Autodesk Inventor part; units mm, degrees
ref_plane "HF-Kabel-DurchlassPunkt" through (-139.5, -56.5, 0) normal (0, -1, 0) x (1, 0, 0)
ref_plane "YZ Plane" through (0, 0, 0) normal (1, 0, 0) x (0, 1, 0)
ref_plane "XZ Plane" through (0, 0, 0) normal (0, 1, 0) x (-1, 0, 0)
sketch "Skizze1" plane through (0, 0, 0) normal (0, 0, 1) x (1, 0, 0)
  line L0 (-149.5, 270.5) -> (149.5, 270.5)
  line L1 (149.5, 270.5) -> (149.5, -270.5)
  line L2 (149.5, -270.5) -> (-149.5, -270.5)
  line L3 (-149.5, -270.5) -> (-149.5, 270.5)
  line L4 (-149.5, 270.5) -> (149.5, -270.5) construction
  line L5 (149.5, 270.5) -> (-149.5, -270.5) construction
  line L6 (-74.75, 270.5) -> (-74.75, -270.5) construction
  line L7 (0, 396.7) -> (0, -381.7) construction
  line L8 (-142.5, 270.5) -> (-142.5, -270.5) construction
  line L9 (-149.5, -162.3) -> (149.5, -162.3) construction
  circle A0 centre (-142.5, -154.8) radius 3.25
  circle A1 centre (-142.5, -169.8) radius 3.25
  line L10 (-222.3, 0) -> (287.3, 0) construction
  circle A2 centre (-142.5, 7.5) radius 3.25
  circle A3 centre (-142.5, -7.5) radius 3.25
  circle A4 centre (-142.5, 154.8) radius 3.25
  circle A5 centre (-142.5, 169.8) radius 3.25
  circle A6 centre (142.5, -154.8) radius 3.25
  circle A7 centre (142.5, -169.8) radius 3.25
  circle A8 centre (142.5, 7.5) radius 3.25
  circle A9 centre (142.5, -7.5) radius 3.25
  circle A10 centre (142.5, 169.8) radius 3.25
  circle A11 centre (142.5, 154.8) radius 3.25
  circle A12 centre (-60, -162.3) radius 2.75
  circle A13 centre (60, -162.3) radius 2.75
  circle A14 centre (-60, 162.3) radius 2.75
  circle A15 centre (60, 162.3) radius 2.75
  line L11 (214.5, 285.5) -> (84.5, 285.5) construction
  line L12 (84.5, 285.5) -> (84.5, 255.5)
  line L13 (84.5, 255.5) -> (214.5, 255.5)
  line L14 (214.5, 255.5) -> (214.5, 285.5) construction
  line L15 (214.5, 285.5) -> (84.5, 255.5) construction
  line L16 (84.5, 285.5) -> (214.5, 255.5) construction
  point P0 (0, 0)
  dimension "d0" = 541
  dimension "d1" = 299
  dimension "d2" = 74.75
  dimension "d3" = 7
  dimension "d4" = 108.2
  dimension "d5" = 6.5
  dimension "d6" = 7.5
  dimension "d7" = 6.5
  dimension "d8" = 7.5
  dimension "d9" = 7.5
  dimension "d10" = 6.5
  dimension "d11" = 5.5
  dimension "d12" = 60
  dimension "d15" = 130
  dimension "d16" = 15
extrude "Extrusion1" add sketch "Skizze1" along normal blind 3
chamfer "Fase1" distance 10 angle 45 4 edges at (149.5, 270.5, 1.5) (149.5, -270.5, 1.5) (-149.5, -270.5, 1.5) (-149.5, 270.5, 1.5)
ref_plane "HF-Kabel-DurchlassPunkt" through (-139.5, -56.5, 0) normal (0, -1, 0) x (1, 0, 0)
sketch "S-AussparungHFKabel" plane through (0, 0, 3) normal (0, 0, 1) x (1, 0, 0)
  line L0 (209.3, -56.5) -> (-209.3, -56.5) construction
  line L1 (-149.5, 260.5) -> (-149.5, -260.5)
  line L2 (-149.5, -75) -> (-129.5, -63.453)
  line L3 (-129.5, -63.453) -> (-129.5, 63.453)
  line L4 (-129.5, 63.453) -> (-149.5, 75)
  line L5 (-129.5, 0) -> (-149.5, 0) construction
  line L6 (-215.9, 0) -> (210.4, 0) construction
  point P0 (0, 0)
  dimension "d21" = 60
  dimension "d22" = 20
  dimension "d23" = 150
extrude "Ex-Kabelaussparung" cut sketch "S-AussparungHFKabel" against normal blind 10
equation "\"d2\" = 0.25 * d1"
equation "\"d4\" = 0.2 * d0"
equation "\"d7\" = d5"
equation "\"d8\" = d6"
equation "\"d9\" = d6"
equation "\"d10\" = d5"
properties part number "enc-BackPanel Unten HF-Durchlass"
Check sheet for the modelled part. Datum: model origin and axes. Units: mm. A direction names the side the tool comes from. Coordinates: 2 decimals unless noted, no trailing zeros. Loops run counter-clockwise (first coordinate to the right, second up) from the corner with the lowest first, then second, coordinate; pieces in that order, holes last. Notation, with made-up numbers: M -16.5,-39 L -10.5,-39 A24 cw -10.5,-10 Z; hole C 29,17.25 d7. An arc over 180 degrees is marked long. Answer as a JSON object with one key per item and string values.
1. Release check for a two-part mould opening along Y. For faces 3 (the flat face through (-2, 4, 3)), 4 (the flat face through (-144, -266, 2)), 5 (the flat face through (-139.36, 69.146, 1.521)), 6 (the flat face through (-145, 265, 2)) record: pulls with the +Y half, pulls with the -Y half, needs draft (parallel to the pull), parting line crosses it, or undercut.
Outcome:
{"face 3": "needs draft", "face 4": "pulls with the -Y half", "face 5": "undercut", "face 6": "pulls with the +Y half"}
2. Scan lines: L1, parallel to Y at x = -60, z = 1.1; L2, parallel to X at y = -154.8, z = 1.95; L3, parallel to X at y = -162.3, z = 1.3. Record each from-to range of solid material in increasing order. Write a range as from..to.
Outcome:
{"L1": "-270.5..-165.05, -159.55..159.55, 165.05..270.5", "L2": "-149.5..-145.75, -139.25..139.25, 145.75..149.5", "L3": "-149.5..-62.75, -57.25..57.25, 62.75..149.5"}
3. Sectioned sample at A-A on z = 1.9. Count the separate pieces of the cut face and the enclosed holes in it, and give its area (3 significant figures).
Outcome:
{"separate pieces": "1", "enclosed holes": "14", "area": "158,000 mm²"}
4. Access from +Z, -Z, +X, -X, +Y, -Y to the whole of each face (thin tool, end or side, straight path). Record for faces 1 (the flat face through (145, 265, 1)), 2 (the flat face through (-139.64, -69.307, 1.521)).
Outcome:
{"face 1": "+Z, -Z, +X, +Y", "face 2": "+Z, -Z, -X"}
5. Sectioned sample at B-B on y = -57.5. Record the cut outline in (x, z).
Outcome:
{"outline": "M -129.5,0 L 149.5,0 L 149.5,3 L -129.5,3 Z"}
6. Depth check by flat-ended pin: P1, Ø4, axis at x = 142.5, y = 7.5, coming from the -Z side. Enter the tip coordinate at first touch or a pass-through.
Outcome:
{"P1": "through"}
